For this review, take the finished solid that the model builds, in its own axes (mm). Coordinates: 2 decimals unless noted, no trailing zeros. Loops run counter-clockwise (first coordinate to the right, second up) from the corner with the lowest first, then second, coordinate; pieces in that order, holes last. Notation, with made-up numbers: (4.25, -22.75) - (51.25, -22.75) arc R30 ccw to (51.25, 1.25) - close; hole circle Ø3 at (14.5, -5). An arc over 180 degrees is marked (long way). Answer as a JSON object with one key per item and string values. Group by question number.
Item 1: Clearance check with a flat-ended pin moving along its axis: pin 1 (3.5 mm diameter, centred on x = 97, z = 4, fed in from +Y). State where the tip first meets the part, or that it passes through.
Item 2: We need section D-D (x = 59). Give the boundary of the cut face in (y, z), then the cut area to 3 significant figures.
Item 3: To check wall thickness, follow line 1 (X direction, y = 30, z = 3.5); line 2 (X direction, y = 6, z = 4); line 3 (Y direction, x = 22.5, z = 3.75). State the ranges of each line that lie inside material, in increasing order.
Item 4: We need section B-B (y = 6.5). Give the boundary of the cut face in (x, z), then the cut area to 3 significant figures.
Item 5: We need section A-A (z = 2). State how many separate pieces and enclosed holes the cut face has, then the cut area to 3 significant figures.
Item 6: We need section C-C (y = 29). Give the boundary of the cut face in (x, z).
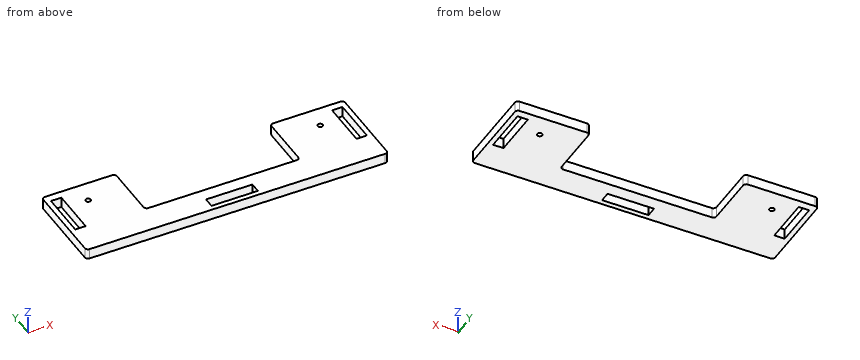
Autodesk Inventor part; units mm, degrees
ref_plane "YZ Plane" through (0, 0, 0) normal (1, 0, 0) x (0, 1, 0)
ref_plane "XZ Plane" through (0, 0, 0) normal (0, 1, 0) x (-1, 0, 0)
ref_plane "XY Plane" through (0, 0, 0) normal (0, 0, 1) x (1, 0, 0)
sketch "Sketch1" plane through (0, 0, 0) normal (0, 0, 1) x (1, 0, 0)
  line L0 (0, 0) -> (195, 0)
  line L1 (195, 0) -> (195, 55)
  line L2 (195, 55) -> (0, 55)
  line L3 (0, 55) -> (0, 0)
  line L4 (3.269, 50) -> (10, 50)
  line L5 (10, 50) -> (10, 20)
  line L6 (10, 20) -> (3.269, 20)
  line L7 (3.269, 20) -> (3.269, 50)
  line L8 (185, 50) -> (191.731, 50)
  line L9 (191.731, 50) -> (191.731, 20)
  line L10 (191.731, 20) -> (185, 20)
  line L11 (185, 20) -> (185, 50)
  line L12 (82.5, 10) -> (112.5, 10)
  line L13 (112.5, 10) -> (112.5, 3.269)
  line L14 (112.5, 3.269) -> (82.5, 3.269)
  line L15 (82.5, 3.269) -> (82.5, 10)
  line L16 (47.5, 55) -> (147.5, 55)
  line L17 (147.5, 55) -> (147.5, 18.269)
  line L18 (147.5, 18.269) -> (47.5, 18.269)
  line L19 (47.5, 18.269) -> (47.5, 55)
  point P0 (3.269, 35)
  point P1 (191.731, 35)
  point P2 (97.5, 18.269)
  point P3 (97.5, 55)
  dimension "d0" = 55
  dimension "d1" = 195
  dimension "d2" = 175
  dimension "d3" = 6.731
  dimension "d4" = 72.5
  dimension "d5" = 72.5
  dimension "d6" = 30
  dimension "d7" = 3.269
  dimension "d8" = 3.269
  dimension "d25" = 10
  dimension "d26" = 10
  dimension "d28" = 36.731
  dimension "d29" = 100
extrude "Extrusion1" add sketch "Sketch1" along normal blind 6.731 contours L3 L2 L19 L18 L17 L1 L0
sketch "Sketch2" plane through (0, 0, 6.731) normal (0, 0, 1) x (1, 0, 0)
  line L0 (10, 50) -> (10, 20)
  line L1 (195, 55) -> (0, 55)
  line L2 (185, 20) -> (185, 50)
  point P0 (22.5, 40.769)
  point P1 (172.5, 40.769)
  dimension "d14" = 150
  dimension "d15" = 14.231
  dimension "d16" = 12.5
  dimension "d30" = 12.5
hole "Hole1" at (22.5, 40.769, 6.731) at (172.5, 40.769, 6.731) direction (0, 0, -1) diameter 3.176 end through all
fillet "Fillet1" radius 2 8 edges at (195, 55, 3.3655) (0, 55, 3.3655) (0, 0, 3.3655) (195, 0, 3.3655) (47.5, 18.269, 3.3655) (47.5, 55, 3.3655) (147.5, 55, 3.3655) (147.5, 18.269, 3.3655)
equation "\"d3\" = THICKB"
equation "\"d4\" = d5"
equation "\"d7\" = d8"
equation "\"d12\" = THICKB"
equation "\"THICKA\" = 3.175"
equation "\"THICKB\" = 6.731"
equation "\"THICKC\" = 12.7"
equation "\"THICKPLY\" = 5"
equation "\"MAGDIA\" = 9.5"
equation "\"BALLDIA\" = 12"
properties part number "Mount_Mega_Back"
Check sheet entries:
{
 "1": {"pin 1": "stops at y = 18.27"},
 "2": {"outline": "(0, 0) - (18.27, 0) - (18.27, 6.73) - (0, 6.73) - close", "area": "123 mm2"},
 "3": {"line 1": "x = 0 to 3.27, 10 to 47.5, 147.5 to 185, 191.73 to 195", "line 2": "x = 0 to 82.5, 112.5 to 195", "line 3": "y = 0 to 39.18, 42.36 to 55"},
 "4": {"outline": "(0, 0) - (82.5, 0) - (82.5, 6.73) - (0, 6.73) - close; (112.5, 0) - (195, 0) - (195, 6.73) - (112.5, 6.73) - close", "area": "1,110 mm2"},
 "5": {"separate pieces": "1", "enclosed holes": "5", "area": "6,430 mm2"},
 "6": {"outline": "(0, 0) - (3.27, 0) - (3.27, 6.73) - (0, 6.73) - close; (10, 0) - (47.5, 0) - (47.5, 6.73) - (10, 6.73) - close; (147.5, 0) - (185, 0) - (185, 6.73) - (147.5, 6.73) - close; (191.73, 0) - (195, 0) - (195, 6.73) - (191.73, 6.73) - close"}
}
